from build123d import *

# Parameters (mm, degrees)
SKETCH_1_W          = 60
SKETCH_1_H          = 77.3
SKETCH_1_R          = 2.25
EXTRUDE_1_DEPTH     = 3
CUT_EXTRUDE_1_DEPTH = 98.899387128
FILLET_2_R          = 1.5
FILLET_3_R          = 5


with BuildPart() as part:
    # 草图1 → 凸台-拉伸1 (new body)
    with BuildSketch(Plane.XY):
        with Locations((30, 38.65)):
            Rectangle(SKETCH_1_W, SKETCH_1_H)
        with Locations((15, 5)):
            Circle(SKETCH_1_R, mode=Mode.SUBTRACT)
        with Locations((45, 5)):
            Circle(SKETCH_1_R, mode=Mode.SUBTRACT)
    extrude(amount=EXTRUDE_1_DEPTH)

    # 草图2 → 切除-拉伸1 (cut, through all)
    with BuildSketch(Plane.XY.offset(3)):
        Polygon((6.498142721, 71.177419939), (25.390067515, 48.791389416), (6.498142721, 27.629402774), align=None)
        Polygon((12.580592965, 71.956095933), (51.165829297, 71.956095933), (31.061830901, 51.954660702), align=None)
        Polygon((54.068167093, 67.235159515), (34.375406047, 47.16148119), (54.068167093, 26.885410871), align=None)
        Polygon((27.938555498, 43.399685415), (6.287330924, 17.986665065), (20.160366982, 7.184410962), (27.938555498, 7.184410962), align=None)
        Polygon((33.25628143, 39.393281631), (33.25628143, 7.119255047), (40.235291957, 7.119255047), (51.165829297, 21.999247226), align=None)
        Polygon((0, 17.3), (11.665719773, 0), (0, 0), align=None)
        Polygon((60, 17.3), (48.617435134, 0), (60, 0), align=None)
    extrude(amount=-CUT_EXTRUDE_1_DEPTH, mode=Mode.SUBTRACT)

    # 圆角2
    fillet_2_edges = [part.edges().sort_by_distance(p)[0] for p in [
        (6.498142721, 27.629402774, 1.5),
        (6.498142721, 71.177419939, 1.5),
        (25.390067515, 48.791389416, 1.5),
        (31.061830901, 51.954660702, 1.5),
        (12.580592965, 71.956095933, 1.5),
        (51.165829297, 71.956095933, 1.5),
        (27.938555498, 43.399685415, 1.5),
        (27.938555498, 7.184410962, 1.5),
        (20.160366982, 7.184410962, 1.5),
        (6.287330924, 17.986665065, 1.5),
        (40.235291957, 7.119255047, 1.5),
        (33.25628143, 7.119255047, 1.5),
        (33.25628143, 39.393281631, 1.5),
        (51.165829297, 21.999247226, 1.5),
        (54.068167093, 67.235159515, 1.5),
        (54.068167093, 26.885410871, 1.5),
        (34.375406047, 47.16148119, 1.5),
    ]]
    fillet(fillet_2_edges, radius=FILLET_2_R)

    # 圆角3
    fillet_3_edges = [part.edges().sort_by_distance(p)[0] for p in [
        (0, 17.3, 1.5),
        (11.665719773, 0, 1.5),
        (0, 77.3, 1.5),
        (60, 17.3, 1.5),
        (60, 77.3, 1.5),
        (48.617435134, 0, 1.5),
    ]]
    fillet(fillet_3_edges, radius=FILLET_3_R)


solid = part.part
Geometry: final body of the model. Coordinates: model frame, mm. A direction names the side the tool comes from. Round coordinates to 2 decimals unless told otherwise and drop trailing zeros. Order: outer loops, then holes, each group sorted by start corner. A loop starts at its lowest first (then second) coordinate and runs counter-clockwise, first axis right, second up. Notation, with made-up numbers: (64.25, 71.5) - (79.25, 71.5) arc R22 ccw to (79.25, 87.5) - close; hole circle Ø4 at (-23.75, -39). An arc over 180 degrees is marked (long way). Write each question's results on one line, items separated by ' | '.
Item 1: First-contact query: pin 1 Ø5 at (x, y) = (45, 5) entering from -Z. Flat tip, straight axial feed; report the tip coordinate or a pass-through.
Completed:
pin 1: z = 0
Item 2: Reachability of faces 1 (the flat face through (30, 0, 1)), 2 (the flat face through (45.47, 14.246, 1.521)) from +Z, -Z, +X, -X, +Y, -Y: full face, straight path, thin tool, end or side. Return the list, or none.
Completed:
face 1: +Z, -Z, +X, -X, -Y | face 2: +Z, -Z
Item 3: Section B-B, the plane y = 32.5. Return the cut outline in (x, z), and give its area (3 significant figures).
Completed:
outline: (0, 0) - (6.5, 0) - (6.5, 3) - (0, 3) - close; (10.85, 0) - (18.65, 0) - (18.65, 3) - (10.85, 3) - close; (27.94, 0) - (33.26, 0) - (33.26, 3) - (27.94, 3) - close; (40.35, 0) - (48.62, 0) - (48.62, 3) - (40.35, 3) - close; (54.07, 0) - (60, 0) - (60, 3) - (54.07, 3) - close | area: 101 mm^2
Item 4: Mould query, pull axis X, two halves, no side actions, for faces 3 (the flat face through (30, 39, 0)), 4 (the cylindrical face through (58.5, 75.87, 1.52)), 5 (the cylindrical face through (14.625, 71.035, 1.479)). Classes: pulls with the +X half, pulls with the -X half, needs draft (parallel to the pull), parting line crosses it, or undercut.
Completed:
face 3: needs draft | face 4: pulls with the +X half | face 5: undercut
Item 5: Section D-D, the plane y = 14.5. Return the cut outline in (x, z).
Completed:
outline: (1.89, 0) - (10.77, 0) - (10.77, 3) - (1.89, 3) - close; (27.94, 0) - (33.26, 0) - (33.26, 3) - (27.94, 3) - close; (45.66, 0) - (58.16, 0) - (58.16, 3) - (45.66, 3) - close
Item 6: Material intervals for line 1 along X through (y, z) = (13, 1.05); line 2 along Y through (x, z) = (50, 2.05); line 3 along Y through (x, z) = (45, 1.25), sorted ascending. Write a range as [from, to].
Completed:
line 1: [2.9, 12.69], [27.94, 33.26], [44.56, 57.17] | line 2: [2.11, 20.41], [23.13, 31.07], [63.09, 77.3] | line 3: [0, 2.75], [7.25, 13.61], [27.99, 36.22], [57.99, 65.82], [71.96, 77.3]
Item 7: Section C-C, the plane x = 23.5. Return the cut outline in (y, z), and give its area (3 significant figures).
Completed:
outline: (0, 0) - (7.18, 0) - (7.18, 3) - (0, 3) - close; (38.19, 0) - (46.67, 0) - (46.67, 3) - (38.19, 3) - close; (51.03, 0) - (60.14, 0) - (60.14, 3) - (51.03, 3) - close; (71.96, 0) - (77.3, 0) - (77.3, 3) - (71.96, 3) - close | area: 90.4 mm^2
Item 8: Section A-A, the plane x = 45. Return the cut outline in (y, z).
Completed:
outline: (0, 0) - (2.75, 0) - (2.75, 3) - (0, 3) - close; (7.25, 0) - (13.61, 0) - (13.61, 3) - (7.25, 3) - close; (27.99, 0) - (36.22, 0) - (36.22, 3) - (27.99, 3) - close; (57.99, 0) - (65.82, 0) - (65.82, 3) - (57.99, 3) - close; (71.96, 0) - (77.3, 0) - (77.3, 3) - (71.96, 3) - close
